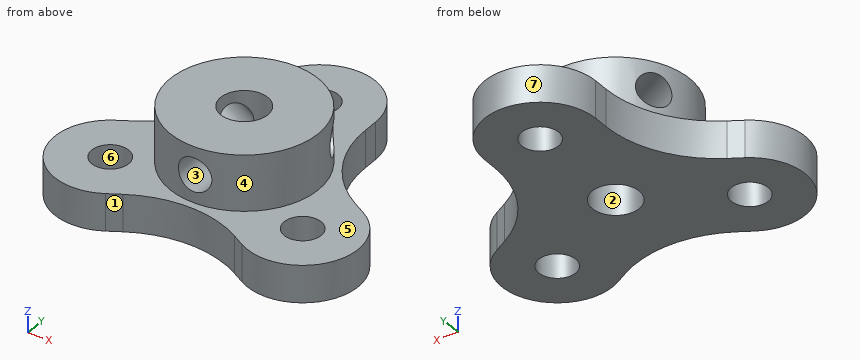
```python
from build123d import *

# Parameters (mm, degrees)
F_1_8_0_1250_DOWEL_HOLE1_D = 3.175
SKETCH6_W                  = 1.4351
SKETCH6_H                  = 21.685653285
CIRPATTERN1_COUNT          = 3
CIRPATTERN2_COUNT          = 3
CUT_EXTRUDE1_START         = -10
SKETCH7_R                  = 15.875
CUT_EXTRUDE1_DEPTH         = 10


with BuildPart() as part:
    # Sketch1 → Revolve1 (revolve)
    with BuildSketch(Plane(origin=(0, 0, 0), x_dir=(0, 0, -1), z_dir=(1, 0, 0)), mode=Mode.PRIVATE) as revolve1_sk:
        Polygon((0, 2.0193), (0, 6.35), (4.7625, 6.35), (4.7625, 15.875), (7.9375, 15.875), (7.9375, 2.0193), align=None)
    revolve(revolve1_sk.sketch.rotate(Axis((0, 0, 0), (0, 0, -1)), 90), axis=Axis((0, 0, 0), (0, 0, -1)))

    # 1/8 (0.1250) Dowel Hole1 (through all)
    with Locations(Plane.XY.offset(-4.7625)):
        with Locations((0, 9.525), (0, 0)):
            f_1_8_0_1250_dowel_hole1 = Hole(F_1_8_0_1250_DOWEL_HOLE1_D / 2)

    # Sketch6 → #6-40 Tapped Hole1 (revolve, cut)
    with BuildSketch(Plane(origin=(0, 0, -2.38125), x_dir=(0, 0, 1), z_dir=(1, 0, 0))):
        with Locations((0.71755, 10.842826643)):
            Rectangle(SKETCH6_W, SKETCH6_H)
    f_6_40_tapped_hole1 = revolve(axis=Axis((0, 6.35, -2.38125), (0, -1, 0)), mode=Mode.SUBTRACT)

    # CirPattern1: #6-40 Tapped Hole1 ×3 about axis
    cirpattern1_axis = Axis((0, 0, 0), (0, 0, 1))
    for i in range(1, CIRPATTERN1_COUNT):
        add(f_6_40_tapped_hole1.rotate(cirpattern1_axis, i * 360 / CIRPATTERN1_COUNT), mode=Mode.SUBTRACT)

    # CirPattern2: 1/8 (0.1250) Dowel Hole1 ×3 about axis
    cirpattern2_axis = Axis((0, 0, 0), (0, 0, 1))
    for i in range(1, CIRPATTERN2_COUNT):
        add(f_1_8_0_1250_dowel_hole1.rotate(cirpattern2_axis, i * 360 / CIRPATTERN2_COUNT), mode=Mode.SUBTRACT)

    # Sketch7 → Cut-Extrude1 (cut)
    with BuildSketch(Plane.XY.offset(-4.7625).offset(CUT_EXTRUDE1_START)):
        Circle(SKETCH7_R)
        with BuildLine():
            ThreePointArc((-4.7625, 9.525), (0, 14.2875), (4.7625, 9.525))
            Line((4.7625, 9.525), (4.7625, 8.248891971))
            ThreePointArc((4.7625, 8.248891971), (6.038608029, 3.486391971), (9.525, 0))
            Line((9.525, 0), (10.630141971, -0.638054014))
            ThreePointArc((10.630141971, -0.638054014), (12.373337957, -7.14375), (5.867641971, -8.886945986))
            Line((5.867641971, -8.886945986), (4.7625, -8.248891971))
            ThreePointArc((4.7625, -8.248891971), (0, -6.972783942), (-4.7625, -8.248891971))
            Line((-4.7625, -8.248891971), (-5.867641971, -8.886945986))
            ThreePointArc((-5.867641971, -8.886945986), (-12.373337957, -7.14375), (-10.630141971, -0.638054014))
            Line((-10.630141971, -0.638054014), (-9.525, 0))
            ThreePointArc((-9.525, 0), (-6.038608029, 3.486391971), (-4.7625, 8.248891971))
            Line((-4.7625, 8.248891971), (-4.7625, 9.525))
        make_face(mode=Mode.SUBTRACT)
    extrude(amount=CUT_EXTRUDE1_DEPTH, mode=Mode.SUBTRACT)


solid = part.part
```
Input: part model. Units: mm. Frame: model coordinates. Face numbers are marked on the shaded views. A direction names the side the tool comes from. Give positions to 0.01 mm unless a question says otherwise; leave off trailing zeros. Order: outer loops, then holes, each group sorted by start corner. A loop starts at its lowest first (then second) coordinate and runs counter-clockwise, first axis right, second up. Notation, with made-up numbers: (81.25, 35.5) - (140.25, 35.5) arc R16 cw to (140.25, 40.5) - close; hole circle Ø1 at (-5.5, 47). An arc over 180 degrees is marked (long way). Put each result on its own line as item: value.
Item 1: Section query A-A, the plane x = 0. Return loops of the section in (y, z), then the cut area to 3 significant figures.
Found:
outline: (-6.97, -7.94) - (-2.02, -7.94) - (-2.02, -3.82) - (-6.35, -3.82) - (-6.35, -4.76) - (-6.97, -4.76) - close; (-6.35, -0.95) - (-2.02, -0.95) - (-2.02, 0) - (-6.35, 0) - close; (2.02, -7.94) - (7.94, -7.94) - (7.94, -4.76) - (6.35, -4.76) - (6.35, 0) - (2.02, 0) - close; (11.11, -7.94) - (14.29, -7.94) - (14.29, -4.76) - (11.11, -4.76) - close
area: 73.4 mm^2
Item 2: Draft query along Y for the marked faces 5, 6 and 7. Return one class per face: +Y half, -Y half, draft (parallel to the pull), parting line (faces both ways), or undercut.
Found:
face 5: draft
face 6: undercut
face 7: +Y half
Item 3: Access query for the marked faces 1, 2, 3 and 4. Directions: +Z, -Z, +X, -X, +Y, -Y. A direction counts if a zero-diameter tool reaches every point of the face in a straight line with its end or side. Return the directions, or none.
Found:
face 1: +Z, -Z, -Y
face 2: +Z, -Z
face 3: -Y
face 4: +Z
Item 4: Contact query for flat-ended pins moving along their axis: pin 1 (2.5 mm diameter, centred on x = -8.25, y = -4.76, fed in from +Z); pin 2 (1.5 mm diameter, centred on x = -8, y = -1, fed in from +Z); pin 3 (1.4 mm diameter, centred on y = 9, z = -6, fed in from -X); pin 4 (4.5 mm diameter, centred on x = 0, z = -2.38, fed in from +Y). Output: stop coordinate, or through.
Found:
pin 1: passes through
pin 2: stops at z = -4.76
pin 3: stops at x = -4.76
pin 4: stops at y = 6.35
Item 5: Ray query, L1, parallel to Y at x = 0, z = -5.95; L2, parallel to Y at x = 0, z = -4.25; L3, parallel to Y at x = 8, z = -6. Return the intervals inside material, ascending. Write a range as from..to.
Found:
L1: y = -6.97..-2.02, 2.02..7.94, 11.11..14.29
L2: y = -6.35..-2.02, 2.02..6.35
L3: y = -9.52..-6.33, -3.19..1.09
Item 6: Section query C-C, the plane z = -2.75. Return loops of the section in (x, y), then the cut area to 3 significant figures.
Found:
outline: (-6.06, 1.9) arc R6.35 ccw to (-1.39, -6.2) - (-1.39, -1.47) arc R2.02 cw to (-1.96, -0.47) - close; (-4.67, 4.3) - (-0.58, 1.93) arc R2.02 cw to (0.58, 1.93) - (4.67, 4.3) arc R6.35 ccw to start; (1.39, -6.2) arc R6.35 ccw to (6.06, 1.9) - (1.96, -0.47) arc R2.02 cw to (1.39, -1.47) - close
area: 76.8 mm^2
Item 7: Section query D-D, the plane z = -5.5. Count the separate pieces of the cut face and the enclosed holes in it, then the cut area to 3 significant figures.
Found:
separate pieces: 1
enclosed holes: 4
area: 318 mm^2
Item 8: Section query B-B, the plane y = -5. Return loops of the section in (x, z).
Found:
outline: (-13.01, -7.94) - (-9.82, -7.94) - (-9.82, -4.76) - (-13.01, -4.76) - close; (-6.68, -7.94) - (6.68, -7.94) - (6.68, -4.76) - (3.91, -4.76) - (3.91, 0) - (-3.91, 0) - (-3.91, -4.76) - (-6.68, -4.76) - close; (9.82, -7.94) - (13.01, -7.94) - (13.01, -4.76) - (9.82, -4.76) - close; hole circle Ø2.87 at (0, -2.38)
